from build123d import *

# Parameters (mm, degrees)
SKETCH1_W             = 50.8
SKETCH1_H             = 25.4
BOSS_EXTRUDE1_DEPTH   = 1.5875
SKETCH2_R             = 0.65
CUT_EXTRUDE1_DEPTH    = 29.442400677
F_4_CLEARANCE_HOLE2_D = 2.9464


with BuildPart() as part:
    # Sketch1 → Boss-Extrude1 (new body)
    with BuildSketch(Plane(origin=(0, 0, 0), x_dir=(1, 0, 0), z_dir=(0, 1, 0))):
        Rectangle(SKETCH1_W, SKETCH1_H)
    extrude(amount=BOSS_EXTRUDE1_DEPTH)

    # Sketch2 → Cut-Extrude1 (cut, through all)
    with BuildSketch(Plane(origin=(0, 1.5875, 0), x_dir=(1, 0, 0), z_dir=(0, 1, 0))):
        with Locations(Location((-2.54, 3.175, 0), (0, 0, 270))):
            Circle(SKETCH2_R)
        with Locations(Location((2.54, 3.175, 0), (0, 0, 270))):
            Circle(SKETCH2_R)
    extrude(amount=-CUT_EXTRUDE1_DEPTH, mode=Mode.SUBTRACT)

    # #4 Clearance Hole2 (through all)
    with Locations(Plane(origin=(0, 1.5875, 0), x_dir=(1, 0, 0), z_dir=(0, 1, 0))):
        with Locations((-12.7, 0), (12.7, 0)):
            Hole(F_4_CLEARANCE_HOLE2_D / 2)


solid = part.part
CAD build for the part. Positions are in the model's coordinates, mm. Coordinates: 2 decimals unless noted, no trailing zeros. Loops run counter-clockwise (first coordinate to the right, second up) from the corner with the lowest first, then second, coordinate; pieces in that order, holes last. Notation, with made-up numbers: (1, 62) - (13, 62) arc R19 cw to (13, 67) - close; hole circle Ø5 at (-13.5, 42.25). An arc over 180 degrees is marked (long way). Write item = value, one per line. Start each with the question number.
Q1. Pull direction Z, two halves, no side cores. Call faces 1 (the cylindrical face through (2.735, 0.805, -2.555)), 2 (the flat face through (0, 1, -12.7)), 3 (the flat face through (0, 0, 0)), 4 (the cylindrical face through (-2.345, 0.805, -2.555)): pulls with the +Z half, pulls with the -Z half, needs draft (parallel to the pull), parting line crosses it, or undercut.
Q2. Cut at A-A, the plane x = 12.7. List the corners of the cut face in (y, z), then the cut area to 3 significant figures.
Q3. Drill centre lines: L1, parallel to Z at x = -12.7, y = 0.4; L2, parallel to Z at x = -11.5, y = 1.4. Where is each one in solid material? Low to high.
Q4. Cut at C-C, the plane x = -2.54. List the corners of the cut face in (y, z) (1 decimal).
Q5. Cut at B-B, the plane z = 0. List the corners of the cut face in (x, y), then the cut area to 3 significant figures.
Q6. Flat gauge pins, fed straight in: pin 1 Ø1 at (x, z) = (2.54, -3.175) entering from +Y; pin 2 Ø3 at (x, z) = (-11.5, 8.5) entering from -Y. Where does each tip first touch, or does it go through?
Computed:
q1.face_1 = undercut
q1.face_2 = pulls with the -Z half
q1.face_3 = needs draft
q1.face_4 = undercut
q2.outline = (0, -12.7) - (1.59, -12.7) - (1.59, -1.47) - (0, -1.47) - close; (0, 1.47) - (1.59, 1.47) - (1.59, 12.7) - (0, 12.7) - close
q2.area = 35.6 mm²
q3.L1 = -12.7 to -1.47, 1.47 to 12.7
q3.L2 = -12.7 to -0.85, 0.85 to 12.7
q4.outline = (0, -12.7) - (1.6, -12.7) - (1.6, -3.8) - (0, -3.8) - close; (0, -2.5) - (1.6, -2.5) - (1.6, 12.7) - (0, 12.7) - close
q5.outline = (-25.4, 0) - (-14.17, 0) - (-14.17, 1.59) - (-25.4, 1.59) - close; (-11.23, 0) - (11.23, 0) - (11.23, 1.59) - (-11.23, 1.59) - close; (14.17, 0) - (25.4, 0) - (25.4, 1.59) - (14.17, 1.59) - close
q5.area = 71.3 mm²
q6.pin_1 = through
q6.pin_2 = 0
